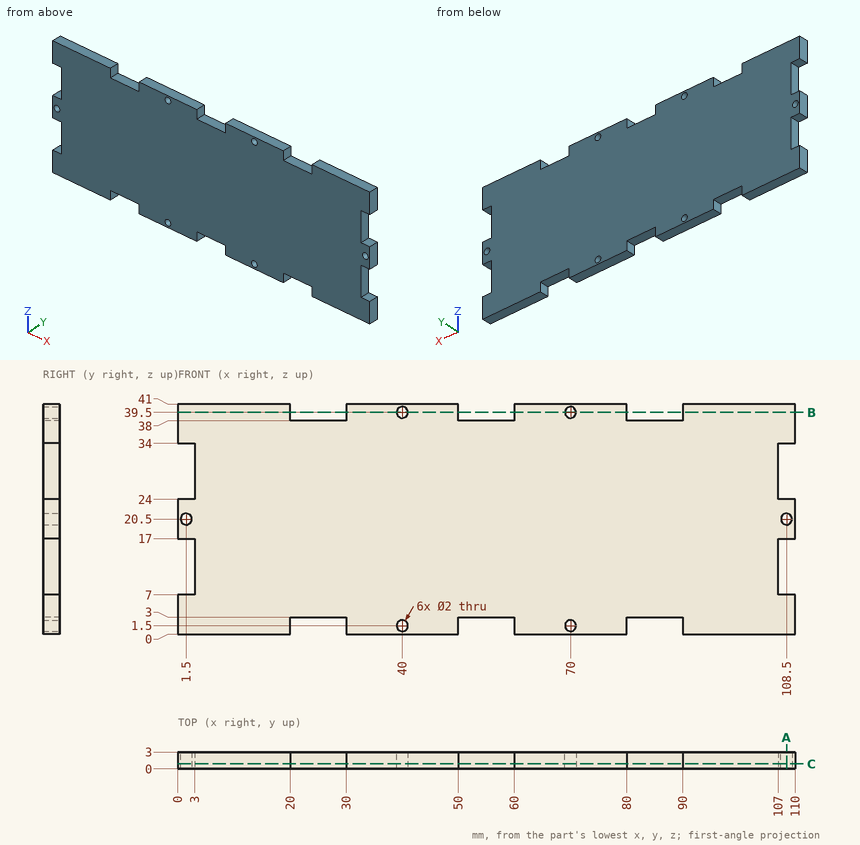
Answer from the drawing. Dimensions are ordinates in mm from the lowest x, y and z of the part. Round coordinates to 2 decimals unless told otherwise and drop trailing zeros. Write each loop counter-clockwise with the first axis right and the second up, starting at its lowest first coordinate (ties: lowest second). Pieces come first, ordered by that corner, then holes. Notation, with made-up numbers: (24.25, 54) - (33.25, 54) arc R23 ccw to (33.25, 86) - close; hole circle Ø5 at (77, 56.25). An arc over 180 degrees is marked (long way). Use a Markdown table: item, result.
(1) The part is cut by section B-B (z = 39.5). Write down the section's boundary in (x, y).
Reported:
| item | result |
|---|---|
| outline | (0, 0) - (20, 0) - (20, 3) - (0, 3) - close; (30, 0) - (39, 0) - (39, 3) - (30, 3) - close; (41, 0) - (50, 0) - (50, 3) - (41, 3) - close; (60, 0) - (69, 0) - (69, 3) - (60, 3) - close; (71, 0) - (80, 0) - (80, 3) - (71, 3) - close; (90, 0) - (110, 0) - (110, 3) - (90, 3) - close |
(2) Straight lines are drawn through the part: line 1 along Z through (x, y) = (40, 1.65); line 2 along Z through (x, y) = (1.5, 1.2); line 3 along X through (y, z) = (0.25, 21). For each, find the intervals that lie inside material, in ascending order. Write a range as [from, to].
Reported:
| item | result |
|---|---|
| line 1 | [0, 0.5], [2.5, 38.5], [40.5, 41] |
| line 2 | [0, 7], [17, 19.5], [21.5, 24], [34, 41] |
| line 3 | [0, 0.63], [2.37, 107.63], [109.37, 110] |
(3) The part is cut by section C-C (y = 0.9). State how many separate pieces and enclosed holes the cut face has, then the cut area to 3 significant figures.
Reported:
| item | result |
|---|---|
| separate pieces | 1 |
| enclosed holes | 6 |
| area | 4,190 mm2 |
(4) Each of these flat-tipped pins is pushed along its axis until it touches: pin 1 Ø0.9 at (y, z) = (1, 11.5) entering from +X; pin 2 Ø0.9 at (y, z) = (1, 26.5) entering from -X; pin 3 Ø3 at (x, z) = (21, 35.5) entering from -Y; pin 4 Ø1 at (x, y) = (58, 1.5) entering from +Z. Where does it stop, or does it pass through?
Reported:
| item | result |
|---|---|
| pin 1 | x = 107 |
| pin 2 | x = 3 |
| pin 3 | y = 0 |
| pin 4 | z = 38 |
(5) The part is cut by section A-A (x = 108.5). Write down the section's boundary in (y, z).
Reported:
| item | result |
|---|---|
| outline | (0, 0) - (3, 0) - (3, 7) - (0, 7) - close; (0, 17) - (3, 17) - (3, 19.5) - (0, 19.5) - close; (0, 21.5) - (3, 21.5) - (3, 24) - (0, 24) - close; (0, 34) - (3, 34) - (3, 41) - (0, 41) - close |
